Read the model definition and answer for the solid it produces. Units are mm, in the model's axes. Face numbers are marked on the shaded views. Coordinates: 2 decimals unless noted, no trailing zeros. Write each loop counter-clockwise with the first axis right and the second up, starting at its lowest first coordinate (ties: lowest second). Pieces come first, ordered by that corner, then holes. Notation, with made-up numbers: (50, 7.5) -> (103, 7.5) arc R26 ccw to (103, 24.5) -> close; hole circle Ø5 at (5, -18). An arc over 180 degrees is marked (long way). Use CSV: the item, a comma, the result in double quotes.
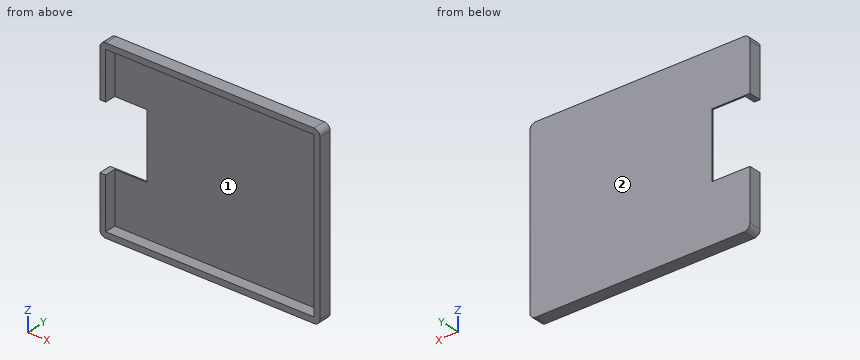
from build123d import *

# Parameters (mm, degrees)
SKETCH2_W           = 74.7
SKETCH2_H           = 59.6
SKETCH2_W_2         = 70.7
SKETCH2_H_2         = 55.6
WALLS_DEPTH         = 3.8
SKETCH3_W           = 59.6
SKETCH3_H           = 0.5
BOSS_EXTRUDE2_DEPTH = 74.7
CUT_EXTRUDE1_REACH  = 93.449
FILLET1_R           = 2


with BuildPart() as part:
    # Sketch2 → walls (new body)
    with BuildSketch(Plane(origin=(0, 15.5, 0), x_dir=(1, 0, 0), z_dir=(0, 1, 0))):
        with Locations((34.35, 26.8)):
            Rectangle(SKETCH2_W, SKETCH2_H)
        with Locations((34.35, 26.8)):
            Rectangle(SKETCH2_W_2, SKETCH2_H_2, mode=Mode.SUBTRACT)
    extrude(amount=WALLS_DEPTH)

    # Sketch3 → Boss-Extrude2 (add)
    with BuildSketch(Plane(origin=(71.7, 0, 0), x_dir=(0, 0, -1), z_dir=(1, 0, 0))):
        with Locations((26.8, 19.55)):
            Rectangle(SKETCH3_W, SKETCH3_H)
    extrude(amount=-BOSS_EXTRUDE2_DEPTH)

    # Sketch4 → Cut-Extrude1 (cut, up to next)
    with BuildSketch(Plane(origin=(0, 15.5, 0), x_dir=(1, 0, 0), z_dir=(0, 1, 0)), mode=Mode.PRIVATE) as cut_extrude1_sk1:
        Polygon((9.95, 37.282193212), (-3, 37.335), (-3, 15.085), (9.95, 15.085), align=None)
    cut_extrude1_tool1 = extrude(cut_extrude1_sk1.sketch, amount=CUT_EXTRUDE1_REACH, mode=Mode.PRIVATE) & part.part
    add(cut_extrude1_tool1.solids().sort_by_distance((3.472436, 15.5, -26.196804))[0], mode=Mode.SUBTRACT)

    # Fillet1
    fillet1_edges = [part.edges().sort_by_distance(p)[0] for p in [
        (71.7, 17.65, -56.6),
        (71.7, 17.65, 3),
        (-3, 17.65, 3),
        (-3, 17.65, -56.6),
    ]]
    fillet(fillet1_edges, radius=FILLET1_R)


solid = part.part
1. A cutting plane is placed at C-C (x = 8.5). Give the vertices of the cut face in (y, z) (3 decimals).
Solutions:
outline,"(15.5, -56.6) -> (19.8, -56.6) -> (19.8, -37.288) -> (19.3, -37.288) -> (19.3, -54.6) -> (15.5, -54.6) -> close; (15.5, 1) -> (19.3, 1) -> (19.3, -15.085) -> (19.8, -15.085) -> (19.8, 3) -> (15.5, 3) -> close"
2. A cutting plane is placed at D-D (x = 33). Give the vertices of the cut face in (y, z), and give its area (3 significant figures).
Solutions:
outline,"(15.5, -56.6) -> (19.8, -56.6) -> (19.8, 3) -> (15.5, 3) -> (15.5, 1) -> (19.3, 1) -> (19.3, -54.6) -> (15.5, -54.6) -> close"
area,"45.0 mm^2"
3. For a pull along X with two mould halves and no side action, classify the marked faces 1 and 2 as pulls with the +X half, pulls with the -X half, needs draft (parallel to the pull), parting line crosses it, or undercut.
Solutions:
face 1,"undercut"
face 2,"needs draft"
4. A cutting plane is placed at B-B (y = 17.05). Give the vertices of the cut face in (x, z) (3 decimals), and give its area (3 significant figures).
Solutions:
outline,"(-3, -54.6) arc R2 ccw to (-1, -56.6) -> (69.7, -56.6) arc R2 ccw to (71.7, -54.6) -> (71.7, 1) arc R2 ccw to (69.7, 3) -> (-1, 3) arc R2 ccw to (-3, 1) -> (-3, -15.085) -> (-1, -15.085) -> (-1, 1) -> (69.7, 1) -> (69.7, -54.6) -> (-1, -54.6) -> (-1, -37.327) -> (-3, -37.335) -> close"
area,"473 mm^2"
5. A cutting plane is placed at A-A (z = -10). Give the vertices of the cut face in (x, y).
Solutions:
outline,"(-3, 15.5) -> (-1, 15.5) -> (-1, 19.3) -> (69.7, 19.3) -> (69.7, 15.5) -> (71.7, 15.5) -> (71.7, 19.8) -> (-3, 19.8) -> close"
6. Each of these flat-tipped pins is pushed along its axis until it touches: pin 1 Ø3 at (x, z) = (50.5, -40) entering from -Y; pin 2 Ø1.9 at (y, z) = (17.5, -33.5) entering from -X. Where does it stop, or does it pass through?
Solutions:
pin 1,"stops at y = 19.3"
pin 2,"stops at x = 69.7"
7. Find the intervals of material crossed by line 1 along Z through (x, y) = (58, 16.1); line 2 along X through (y, z) = (17.8, -50.5); line 3 along X through (y, z) = (16.9, -33.5), in increasing order.
Solutions:
line 1,"z = -56.6 to -54.6, 1 to 3"
line 2,"x = -3 to -1, 69.7 to 71.7"
line 3,"x = 69.7 to 71.7"
